Read the model definition and answer for the solid it produces. Units are mm, in the model's axes. Face numbers are marked on the shaded views. A direction names the side the tool comes from. Round coordinates to 2 decimals unless told otherwise and drop trailing zeros. Write each loop counter-clockwise with the first axis right and the second up, starting at its lowest first coordinate (ties: lowest second). Pieces come first, ordered by that corner, then holes. Notation, with made-up numbers: (-39, -33.5) -> (-9, -33.5) arc R35 ccw to (-9, 1.5) -> close; hole circle Ø7 at (-23.5, -38). An arc over 180 degrees is marked (long way). Return JSON: item names as keys, results as strings.
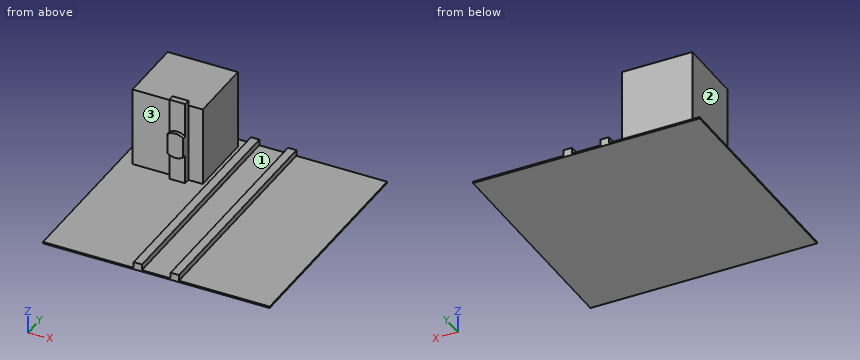
from build123d import *

# Parameters (mm, degrees)
SKETCH1_W           = 1500
SKETCH1_H           = 1500
BOSS_EXTRUDE1_DEPTH = 10
SKETCH2_W           = 465
SKETCH2_H           = 450
BOSS_EXTRUDE2_DEPTH = 525
SKETCH3_W           = 105
SKETCH3_H           = 557.5
BOSS_EXTRUDE3_DEPTH = 40
BOSS_EXTRUDE4_DEPTH = 65
SKETCH4_W           = 55
SKETCH4_H           = 1500
BOSS_EXTRUDE5_DEPTH = 40


with BuildPart() as part:
    # Sketch1 → Boss-Extrude1 (new body)
    with BuildSketch(Plane.XY):
        with Locations((-750, 750)):
            Rectangle(SKETCH1_W, SKETCH1_H)
    extrude(amount=BOSS_EXTRUDE1_DEPTH)

    # Sketch2 → Boss-Extrude2 (add)
    with BuildSketch(Plane.XY.offset(10)):
        with Locations((-1182.5, 1205)):
            Rectangle(SKETCH2_W, SKETCH2_H)
    extrude(amount=BOSS_EXTRUDE2_DEPTH)

    # Sketch3 → Boss-Extrude3 (add)
    with BuildSketch(Plane.XZ.offset(-980)):
        with Locations((-1098.62392171, 288.75)):
            Rectangle(SKETCH3_W, SKETCH3_H)
    extrude(amount=BOSS_EXTRUDE3_DEPTH)

    # Sketch3<3> → Boss-Extrude4 (add)
    with BuildSketch(Plane.XZ.offset(-980)):
        with BuildLine():
            ThreePointArc((-1046.12392171, 339.348709786), (-1098.62392171, 357.5), (-1151.12392171, 339.348709786))
            Line((-1151.12392171, 339.348709786), (-1151.12392171, 205.651290214))
            ThreePointArc((-1151.12392171, 205.651290214), (-1098.62392171, 187.5), (-1046.12392171, 205.651290214))
            Line((-1046.12392171, 205.651290214), (-1046.12392171, 339.348709786))
        make_face()
    extrude(amount=BOSS_EXTRUDE4_DEPTH)

    # Sketch4 → Boss-Extrude5 (add)
    with BuildSketch(Plane.XY.offset(10)):
        with Locations((-872.5, 750)):
            Rectangle(SKETCH4_W, SKETCH4_H)
        with Locations((-627.5, 750)):
            Rectangle(SKETCH4_W, SKETCH4_H)
    extrude(amount=BOSS_EXTRUDE5_DEPTH)


solid = part.part
Item 1: Section A-A (y = 1078) is taken. Give the vertices of the cut face in (x, z), then the cut area to 3 significant figures.
Worked answers:
{"outline": "(-1500, 0) -> (0, 0) -> (0, 10) -> (-600, 10) -> (-600, 50) -> (-655, 50) -> (-655, 10) -> (-845, 10) -> (-845, 50) -> (-900, 50) -> (-900, 10) -> (-950, 10) -> (-950, 535) -> (-1415, 535) -> (-1415, 10) -> (-1500, 10) -> close", "area": "264,000 mm2"}
Item 2: Straight lines are drawn through the part: L1, parallel to Z at x = -585.5, y = 1383; L2, parallel to X at y = 951, z = 117.5; L3, parallel to X at y = 1296.5, z = 349. For each, find the intervals that lie inside material, in ascending order. Write a range as [from, to].
Worked answers:
{"L1": "z = [0, 10]", "L2": "x = [-1151.12, -1046.12]", "L3": "x = [-1415, -950]"}
Item 3: Flat-ended cylindrical pins translate along their axes: pin 1 (3 mm diameter, centred on x = -1028.5, z = 210.5, fed in from -Y); pin 2 (20 mm diameter, centred on y = 1032, z = 25.5, fed in from -X); pin 3 (1 mm diameter, centred on y = 1085.5, z = 252.5, fed in from +X). Find the tip coordinate at first contact, or state that the pin passes through.
Worked answers:
{"pin 1": "stops at y = 980", "pin 2": "stops at x = -1415", "pin 3": "stops at x = -950"}
Item 4: Section D-D (y = 330) is taken. Give the vertices of the cut face in (x, z), then the cut area to 3 significant figures.
Worked answers:
{"outline": "(-1500, 0) -> (0, 0) -> (0, 10) -> (-600, 10) -> (-600, 50) -> (-655, 50) -> (-655, 10) -> (-845, 10) -> (-845, 50) -> (-900, 50) -> (-900, 10) -> (-1500, 10) -> close", "area": "19,400 mm2"}
Item 5: A tool of negligible diameter and unlimited length cuts with its end or side. For the marked faces 1, 2 and 3, from which of +Z, -Z, +X, -X, +Y, -Y can it reach the whole face along a straight path? Write none if from no direction.
Worked answers:
{"face 1": "+Z, +Y, -Y", "face 2": "+Z, -X, +Y, -Y", "face 3": "+Z, -X, -Y"}
Item 6: Section C-C (z = 435) is taken. Give the vertices of the cut face in (x, y).
Worked answers:
{"outline": "(-1415, 980) -> (-1151.12, 980) -> (-1151.12, 940) -> (-1046.12, 940) -> (-1046.12, 980) -> (-950, 980) -> (-950, 1430) -> (-1415, 1430) -> close"}
Item 7: Section B-B (x = -1362.5) is taken. Give the vertices of the cut face in (y, z), then the cut area to 3 significant figures.
Worked answers:
{"outline": "(0, 0) -> (1500, 0) -> (1500, 10) -> (1430, 10) -> (1430, 535) -> (980, 535) -> (980, 10) -> (0, 10) -> close", "area": "251,000 mm2"}
